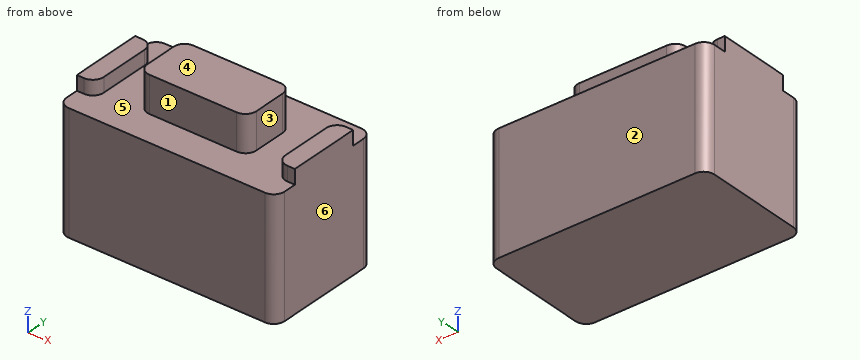
from build123d import *

# Parameters (mm, degrees)
SKETCH_W     = 6
SKETCH_H     = 3.3
PAD_DEPTH    = 3.3
SKETCH001_W  = 3
SKETCH001_H  = 1.5
PAD001_DEPTH = 4.3
SKETCH002_W  = 0.5
SKETCH002_H  = 2
PAD002_DEPTH = 3.7
FILLET_R     = 0.3


with BuildPart() as part:
    # Sketch → Pad (new body)
    with BuildSketch(Plane.XY):
        Rectangle(SKETCH_W, SKETCH_H)
    extrude(amount=PAD_DEPTH)

    # Sketch001 → Pad001 (join)
    with BuildSketch(Plane.XY):
        Rectangle(SKETCH001_W, SKETCH001_H)
    extrude(amount=PAD001_DEPTH)

    # Sketch002 → Pad002 (join)
    with BuildSketch(Plane.XY):
        with Locations((-2.75, 0)):
            Rectangle(SKETCH002_W, SKETCH002_H)
        with Locations((2.75, 0)):
            Rectangle(SKETCH002_W, SKETCH002_H)
    extrude(amount=PAD002_DEPTH)

    # Fillet
    fillet_edges = [part.edges().sort_by_distance(p)[0] for p in [
        (3, -1.65, 1.65),
        (-3, -1.65, 1.65),
        (3, 1.65, 1.65),
        (1.5, -0.75, 3.8),
        (1.5, 0.75, 3.8),
        (2.5, -1, 3.5),
        (-2.5, -1, 3.5),
        (-2.5, 1, 3.5),
        (-1.5, -0.75, 3.8),
        (2.5, 1, 3.5),
        (-1.5, 0.75, 3.8),
        (-3, 1.65, 1.65),
    ]]
    fillet(fillet_edges, radius=FILLET_R)


solid = part.part
The listing builds one solid part. Answer for the finished solid, in the listing's coordinates (mm). Face numbers are marked on the shaded views. A direction names the side the tool comes from. Round coordinates to 2 decimals unless told otherwise and drop trailing zeros. Order: outer loops, then holes, each group sorted by start corner. A loop starts at its lowest first (then second) coordinate and runs counter-clockwise, first axis right, second up. Notation, with made-up numbers: (-17, 23) -> (39, 23) arc R15 cw to (39, 41) -> close; hole circle Ø9 at (-2.5, 13). An arc over 180 degrees is marked (long way). Write each question's results on one line, items separated by ' | '. Start each with the question number.
Q1. Find section D-D (x = -2.4). Determine the outline of the cut face in (y, z).
Q2. Which of the six approach directions +Z, -Z, +X, -X, +Y, -Y give full straight-line access (tool end or side, diameter ignored) to the marked faces 1, 2 and 3?
Q3. The mould has two halves that part along X. Classify the marked faces 4, 5 and 6: pulls with the +X half, pulls with the -X half, needs draft (parallel to the pull), parting line crosses it, or undercut.
Q4. Find section C-C (y = 0.25). Determine the outline of the cut face in (x, z).
Q5. Find section A-A (z = 3.55). Determine the outline of the cut face in (x, y), then the cut area to 3 significant figures.
Q6. Find section B-B (x = -1.1). Determine the outline of the cut face in (y, z), then the cut area to 3 significant figures.
Q7. Straight lines are drawn through the part: probe 1 along Z at (x, y) = (1.1, 1.2); probe 2 along Y at (x, z) = (0, 4.15); probe 3 along X at (y, z) = (0.15, 4.1). For each, find the intervals that lie inside material, in ascending order. Write a range as from..to.
Q8. This flat-tipped pin is pushed along its axis until it touches: pin 1 (0.5 mm diameter, centred on x = 0.5, z = 4, fed in from -Y). Where does it stop, or does it pass through?
Worked answers:
1) outline: (-1.65, 0) -> (1.65, 0) -> (1.65, 3.3) -> (-1.65, 3.3) -> close
2) face 1: +Z, -Y | face 2: +Z, -Z, +X, -X, +Y | face 3: +Z, +Y, -Y
3) face 4: needs draft | face 5: undercut | face 6: pulls with the +X half
4) outline: (-3, 0) -> (3, 0) -> (3, 3.7) -> (2.5, 3.7) -> (2.5, 3.3) -> (1.5, 3.3) -> (1.5, 4.3) -> (-1.5, 4.3) -> (-1.5, 3.3) -> (-2.5, 3.3) -> (-2.5, 3.7) -> (-3, 3.7) -> close
5) outline: (-3, -1) -> (-2.8, -1) arc R0.3 ccw to (-2.5, -0.7) -> (-2.5, 0.7) arc R0.3 ccw to (-2.8, 1) -> (-3, 1) -> close; (-1.5, -0.45) arc R0.3 ccw to (-1.2, -0.75) -> (1.2, -0.75) arc R0.3 ccw to (1.5, -0.45) -> (1.5, 0.45) arc R0.3 ccw to (1.2, 0.75) -> (-1.2, 0.75) arc R0.3 ccw to (-1.5, 0.45) -> close; (2.5, -0.7) arc R0.3 ccw to (2.8, -1) -> (3, -1) -> (3, 1) -> (2.8, 1) arc R0.3 ccw to (2.5, 0.7) -> close | area: 6.35 mm2
6) outline: (-1.65, 0) -> (1.65, 0) -> (1.65, 3.3) -> (0.75, 3.3) -> (0.75, 4.3) -> (-0.75, 4.3) -> (-0.75, 3.3) -> (-1.65, 3.3) -> close | area: 12.4 mm2
7) probe 1: z = 0..3.3 | probe 2: y = -0.75..0.75 | probe 3: x = -1.5..1.5
8) pin 1: stops at y = -0.75
